Verification items for the finished model (mm, model axes). Face numbers are marked on the shaded views. A direction names the side the tool comes from. Give positions to 0.01 mm unless a question says otherwise; leave off trailing zeros. Loops run counter-clockwise (first coordinate to the right, second up) from the corner with the lowest first, then second, coordinate; pieces in that order, holes last. Notation, with made-up numbers: (-18.5, 53) - (-6.5, 53) arc R34 ccw to (-6.5, 87) - close; hole circle Ø6 at (80.25, 75.5). An arc over 180 degrees is marked (long way). Use one line per item in the form item = value.
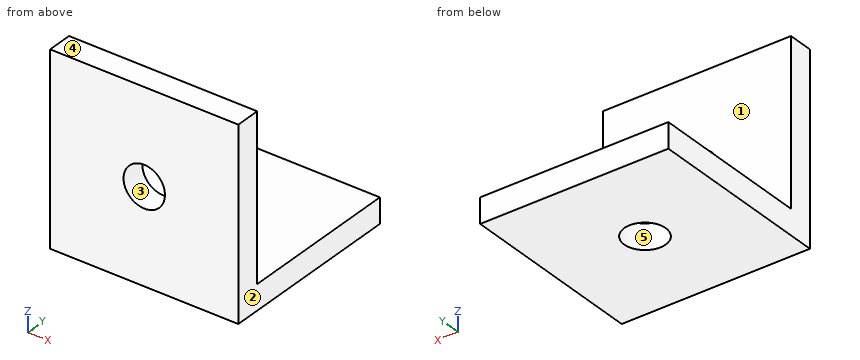
```python
from build123d import *

# Parameters (mm, degrees)
F1_DEPTH = 15
F3_D     = 3.3
F5_D     = 3.3


with BuildPart() as f1:
    # F0 (on Right) → F1 (new body)
    with BuildSketch(Plane.YZ):
        Polygon((0, 15), (0, 0), (15, 0), (15, 2), (2, 2), (2, 15), align=None)
    extrude(amount=F1_DEPTH)

    # F3 (through all)
    with Locations(Plane(origin=(0, 0, 0), x_dir=(1, 0, 0), z_dir=(0, 0, -1))):
        with Locations((7.5, -7.5)):
            Hole(F3_D / 2)

    # F5 (through all)
    with Locations(Plane.XZ):
        with Locations((7.5, 7.5)):
            Hole(F5_D / 2)


solid = f1.part
```
1. Section check B-B, the plane y = 7.5. Record the cut outline in (x, z).
Result set:
outline = (0, 0) - (5.85, 0) - (5.85, 2) - (0, 2) - close; (9.15, 0) - (15, 0) - (15, 2) - (9.15, 2) - close
2. Section check A-A, the plane x = 7.5. Record the cut outline in (y, z).
Result set:
outline = (0, 0) - (5.85, 0) - (5.85, 2) - (2, 2) - (2, 5.85) - (0, 5.85) - close; (0, 9.15) - (2, 9.15) - (2, 15) - (0, 15) - close; (9.15, 0) - (15, 0) - (15, 2) - (9.15, 2) - close
3. Section check D-D, the plane x = 2.75. Record the cut outline in (y, z).
Result set:
outline = (0, 0) - (15, 0) - (15, 2) - (2, 2) - (2, 15) - (0, 15) - close
4. Depth check by flat-ended pin: pin 1 Ø1.5 at (x, z) = (7.5, 10) entering from +Y; pin 2 Ø4 at (x, y) = (8.5, 6) entering from +Z. Enter the tip coordinate at first touch or a pass-through.
Result set:
pin_1 = 2
pin_2 = 2
5. Tool access check on the marked faces 1 and 2. Record the directions out of +Z, -Z, +X, -X, +Y, -Y that give a thin tool (end or side, any length) a straight path to the whole face; none if there is none.
Result set:
face_1 = +Z, +X, -X, +Y
face_2 = +Z, -Z, +X, +Y, -Y
6. Scan lines: probe 1 along Y at (x, z) = (7.5, 1); probe 2 along Z at (x, y) = (1, 13.5). Record each from-to range of solid material in increasing order.
Result set:
probe_1 = 0 to 5.85, 9.15 to 15
probe_2 = 0 to 2
7. Draft check along Z on the marked faces 3, 4 and 5. Enter one of: released by +Z, released by -Z, zero draft, split by the parting line, or undercut.
Result set:
face_3 = undercut
face_4 = released by +Z
face_5 = zero draft
